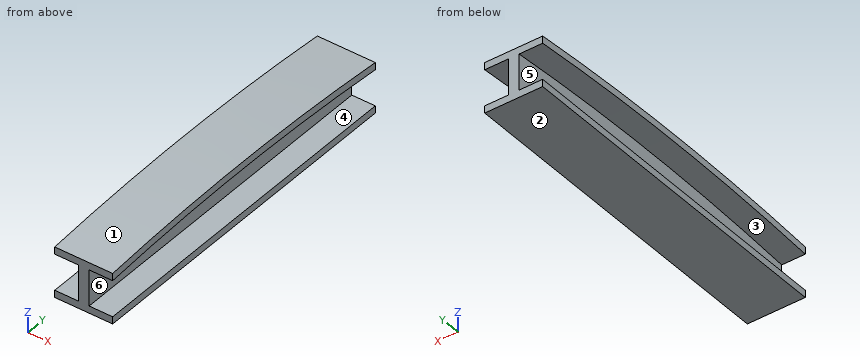
```python
from build123d import *

# Parameters (mm, degrees)
F0_W     = 304.8
F0_H     = 6.35
F1_DEPTH = 50.8
F3_DEPTH = 0.8125
F5_DEPTH = 20.6502


# Not quite as in the source:
# - a pattern or mirror of a feature is missing from the dataset's text; its kind, count and spacing are read off the source's solid


with BuildPart() as f1:
    # F0 (on Right) → F1 (new body)
    with BuildSketch(Plane.YZ):
        with BuildLine():
            Line((-304.8, 6.35), (0, 6.35))
            Line((0, 6.35), (0, 38.1))
            ThreePointArc((0, 38.1), (-152.4, 44.45), (-304.8, 38.1))
            Line((-304.8, 38.1), (-304.8, 6.35))
        make_face()
        with BuildLine():
            ThreePointArc((-304.8, 38.1), (-152.4, 44.45), (0, 38.1))
            Line((0, 38.1), (0, 44.45))
            ThreePointArc((0, 44.45), (-152.4, 50.8), (-304.8, 44.45))
            Line((-304.8, 44.45), (-304.8, 38.1))
        make_face()
        with Locations((-152.4, 3.175)):
            Rectangle(F0_W, F0_H)
    extrude(amount=F1_DEPTH)

    # F2 (on face) → F3 (cut)
    with BuildSketch(Plane.YZ.offset(50.8)):
        with BuildLine():
            Line((0, 6.35), (0, 38.1))
            ThreePointArc((0, 38.1), (-152.4, 44.45), (-304.8, 38.1))
            Line((-304.8, 38.1), (-304.8, 6.35))
            Line((-304.8, 6.35), (0, 6.35))
        make_face()
    extrude(amount=-F3_DEPTH, mode=Mode.SUBTRACT)

    # F4 (on face) → F5 (cut)
    with BuildSketch(Plane(origin=(0, 0, 0), x_dir=(0, -1, 0), z_dir=(-1, 0, 0))):
        with BuildLine():
            Line((304.8, 6.35), (304.8, 38.1))
            ThreePointArc((304.8, 38.1), (152.4, 44.45), (0, 38.1))
            Line((0, 38.1), (0, 6.35))
            Line((0, 6.35), (304.8, 6.35))
        make_face()
    f5 = extrude(amount=-F5_DEPTH, mode=Mode.SUBTRACT)

    # F5_copies: F5 across plane
    add(f5.mirror(Plane(origin=(25.40635, 0, 0), x_dir=(0, 0, 1), z_dir=(1, 0, 0))), mode=Mode.SUBTRACT)


solid = f1.part
```
Input: part model. Units: mm. Frame: model coordinates. Face numbers are marked on the shaded views. A direction names the side the tool comes from. Round coordinates to 2 decimals unless told otherwise and drop trailing zeros. Loops run counter-clockwise (first coordinate to the right, second up) from the corner with the lowest first, then second, coordinate; pieces in that order, holes last.
1) Set-up query: the marked faces 4, 5 and 6. Return all of +Z, -Z, +X, -X, +Y, -Y with unobstructed straight access to the full face (end or side cutting, diameter ignored); none if empty.
Ans:
face 4: +X, +Y, -Y
face 5: -X
face 6: +X
2) Section query A-A on x = 18. Return the cut outline in (y, z) (3 decimals), plus the area to 3 significant figures.
Ans:
outline: (-304.8, 0) - (0, 0) - (0, 6.35) - (-304.8, 6.35) - close; (-304.8, 38.1) arc R1831.975 cw to (0, 38.1) - (0, 44.45) arc R1831.975 ccw to (-304.8, 44.45) - close
area: 3,870 mm2
3) Section query C-C on z = 32. Return the cut outline in (x, y), plus the area to 3 significant figures.
Ans:
outline: (20.65, -304.8) - (30.16, -304.8) - (30.16, 0) - (20.65, 0) - close
area: 2,900 mm2
4) Section query B-B on y = -98.5. Return the cut outline in (x, z), plus the area to 3 significant figures.
Ans:
outline: (0, 0) - (50.8, 0) - (50.8, 6.35) - (30.16, 6.35) - (30.16, 43.66) - (50.8, 43.66) - (50.8, 50.01) - (0, 50.01) - (0, 43.66) - (20.65, 43.66) - (20.65, 6.35) - (0, 6.35) - close
area: 1,000 mm2
5) Section query D-D on y = -138. Return the cut outline in (x, z).
Ans:
outline: (0, 0) - (50.8, 0) - (50.8, 6.35) - (30.16, 6.35) - (30.16, 44.39) - (50.8, 44.39) - (50.8, 50.74) - (0, 50.74) - (0, 44.39) - (20.65, 44.39) - (20.65, 6.35) - (0, 6.35) - close
6) Pin query (flat end, axial travel): pin 1 (12 mm diameter, centred on y = -121, z = 31.5, fed in from -X); pin 2 (10.5 mm diameter, centred on x = 45, y = -139, fed in from +Z). Return the tip coordinate at first contact, or that it passes through.
Ans:
pin 1: stops at x = 20.65
pin 2: stops at z = 50.78
7) Pull-direction query (Y, two-part tool) for the marked faces 1, 2 and 3; classes: released by +Y, released by -Y, zero draft, split by the parting line, or undercut.
Ans:
face 1: split by the parting line
face 2: zero draft
face 3: undercut
8) Material intervals for line 1 (Z direction, x = 15.5, y = -165); line 2 (X direction, y = -17.5, z = 7); line 3 (Z direction, x = 12.5, y = -252.5), sorted ascending.
Ans:
line 1: z = 0 to 6.35, 44.41 to 50.76
line 2: x = 20.65 to 30.16
line 3: z = 0 to 6.35, 41.71 to 48.06
